Design review of the part built by this model. Coordinates are the model's own, in mm. Coordinates: 2 decimals unless noted, no trailing zeros. Write each loop counter-clockwise with the first axis right and the second up, starting at its lowest first coordinate (ties: lowest second). Pieces come first, ordered by that corner, then holes. Notation, with made-up numbers: (67, 69) -> (83, 69) arc R19 ccw to (83, 97) -> close; hole circle Ø5 at (-6, 42). An arc over 180 degrees is marked (long way). Answer in a Markdown table with one row per item. Add a question column.
Item 1: Take a section at D-D, the plane x = -7.5. Write out the cut boundary in (y, z), and give its area (3 significant figures).
Item 2: Take a section at B-B, the plane x = -30. Write out the cut boundary in (y, z), and give its area (3 significant figures).
Item 3: Take a section at A-A, the plane z = 0. Write out the cut boundary in (x, y), and give its area (3 significant figures).
Item 4: To check wall thickness, follow line 1 (X direction, y = 2.65, z = 0); line 2 (X direction, y = 4.3, z = 0); line 3 (X direction, y = 2.5, z = 21). State the ranges of each line that lie inside material, in increasing order.
Item 5: Take a section at C-C, the plane y = 2. Write out the cut boundary in (x, z).
Item 6: Clearance check with flat-ended pins moving along their axes: P1, Ø3.5, axis at x = 30, z = -15, coming from the +Y side; P2, Ø1.5, axis at x = -4.5, y = 1.5, coming from the +Z side; P3, Ø5, axis at x = -7.5, z = 0, coming from the -Y side. State where each tip first meets the part, or that it passes through.
from build123d import *

# Parameters (mm, degrees)
SKETCH1_R           = 2
BOSS_EXTRUDE1_DEPTH = 5
SKETCH2_R           = 4
CUT_EXTRUDE1_DEPTH  = 4
SKETCH2_4_R         = 2
CUT_EXTRUDE2_DEPTH  = 48.434164903


with BuildPart() as part:
    # Sketch1 → Boss-Extrude1 (new body)
    with BuildSketch(Plane(origin=(0, 0, 0), x_dir=(1, 0, 0), z_dir=(0, 1, 0))):
        Polygon((-40, -25), (-17.5, -25), (-17.5, -18), (17.5, -18), (17.5, -25), (40, -25), (40, 25), (-40, 25), align=None)
        with Locations(Location((-30, -15, 0), (0, 0, 270))):
            Circle(SKETCH1_R, mode=Mode.SUBTRACT)
        with Locations(Location((30, -15, 0), (0, 0, 270))):
            Circle(SKETCH1_R, mode=Mode.SUBTRACT)
        with Locations(Location((-30, 15, 0), (0, 0, 270))):
            Circle(SKETCH1_R, mode=Mode.SUBTRACT)
        with Locations(Location((30, 15, 0), (0, 0, 270))):
            Circle(SKETCH1_R, mode=Mode.SUBTRACT)
    extrude(amount=BOSS_EXTRUDE1_DEPTH)

    # Sketch2 → Cut-Extrude1 (cut)
    with BuildSketch(Plane.XZ):
        with Locations(Location((-7.5, 0, 0), (0, 0, 270))):
            Circle(SKETCH2_R)
        with Locations(Location((7.5, 0, 0), (0, 0, 270))):
            Circle(SKETCH2_R)
    extrude(amount=-CUT_EXTRUDE1_DEPTH, mode=Mode.SUBTRACT)

    # Sketch2_4 → Cut-Extrude2 (cut, through all)
    with BuildSketch(Plane.XZ):
        with Locations(Location((-7.5, 0, 0), (0, 0, 270))):
            Circle(SKETCH2_4_R)
        with Locations(Location((7.5, 0, 0), (0, 0, 270))):
            Circle(SKETCH2_4_R)
    extrude(amount=-CUT_EXTRUDE2_DEPTH, mode=Mode.SUBTRACT)


solid = part.part
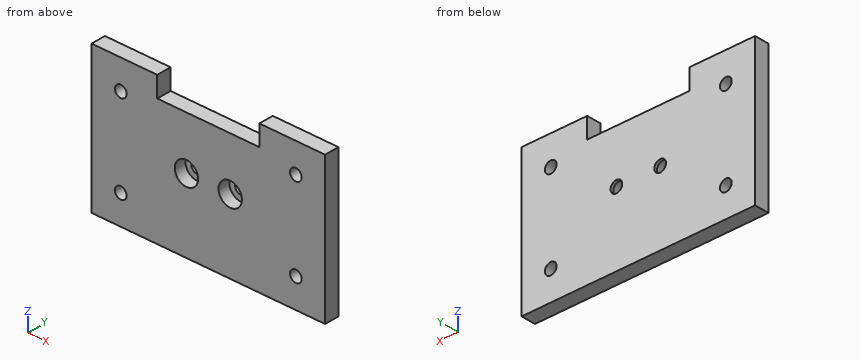
Answers:
| question | item | result |
|---|---|---|
| 1 | outline | (0, -25) -> (5, -25) -> (5, -2) -> (4, -2) -> (4, -4) -> (0, -4) -> close; (0, 4) -> (4, 4) -> (4, 2) -> (5, 2) -> (5, 18) -> (0, 18) -> close |
| 1 | area | 179 mm^2 |
| 2 | outline | (0, -25) -> (5, -25) -> (5, -17) -> (0, -17) -> close; (0, -13) -> (5, -13) -> (5, 13) -> (0, 13) -> close; (0, 17) -> (5, 17) -> (5, 25) -> (0, 25) -> close |
| 2 | area | 210 mm^2 |
| 3 | outline | (-40, 0) -> (-11.5, 0) -> (-11.5, 4) -> (-9.5, 4) -> (-9.5, 5) -> (-40, 5) -> close; (-5.5, 4) -> (-3.5, 4) -> (-3.5, 0) -> (3.5, 0) -> (3.5, 4) -> (5.5, 4) -> (5.5, 5) -> (-5.5, 5) -> close; (9.5, 4) -> (11.5, 4) -> (11.5, 0) -> (40, 0) -> (40, 5) -> (9.5, 5) -> close |
| 3 | area | 328 mm^2 |
| 4 | line 1 | x = -40 to -11.5, -3.5 to 3.5, 11.5 to 40 |
| 4 | line 2 | x = -40 to -9.5, -5.5 to 5.5, 9.5 to 40 |
| 4 | line 3 | x = -40 to -17.5, 17.5 to 40 |
| 5 | outline | (-40, -25) -> (40, -25) -> (40, 25) -> (17.5, 25) -> (17.5, 18) -> (-17.5, 18) -> (-17.5, 25) -> (-40, 25) -> close; hole circle Ø4 at (-30, -15); hole circle Ø4 at (-30, 15); hole circle Ø8 at (-7.5, 0); hole circle Ø8 at (7.5, 0); hole circle Ø4 at (30, -15); hole circle Ø4 at (30, 15) |
| 6 | P1 | passes through |
| 6 | P2 | stops at z = 18 |
| 6 | P3 | stops at y = 4 |
